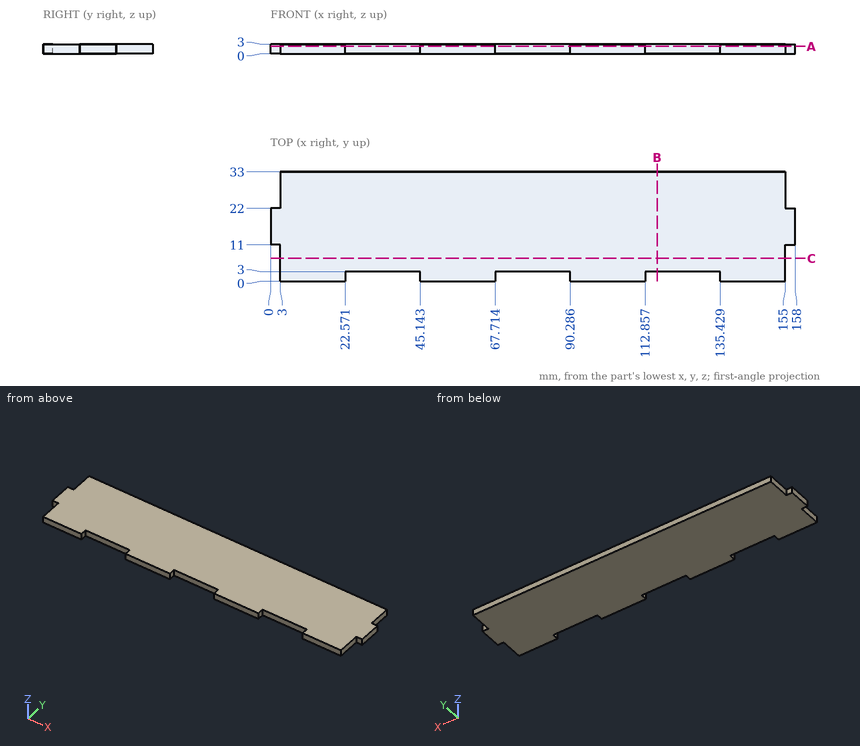
Drawing for the job (mm, zero at the part's lowest x, y, z). Round coordinates to 2 decimals unless told otherwise and drop trailing zeros. Order: outer loops, then holes, each group sorted by start corner. A loop starts at its lowest first (then second) coordinate and runs counter-clockwise, first axis right, second up. Notation, with made-up numbers: (87.5, 54.25) -> (96.5, 54.25) arc R13 cw to (96.5, 68.25) -> close; hole circle Ø9 at (81, 28.25). An arc over 180 degrees is marked (long way). Put each result on its own line as item: value.
Q1. Band-saw the part on C-C (y = 7). Give the cut face in (x, z).
From the geometry:
outline: (3, 0) -> (155, 0) -> (155, 3) -> (3, 3) -> close
Q2. Wall check: line 1 (X direction, y = 2, z = 2.8) (1 decimal); line 2 (Y direction, x = 85.5, z = 2); line 3 (X direction, y = 7, z = 2.6). Give the ranges that are in metal, low to high. Write a range as [from, to].
From the geometry:
line 1: x = [3, 22.6], [45.1, 67.7], [90.3, 112.9], [135.4, 155]
line 2: y = [3, 33]
line 3: x = [3, 155]
Q3. Band-saw the part on A-A (z = 2.3). Give the cut face in (x, y) (1 decimal), and give its area (3 significant figures).
From the geometry:
outline: (0, 11) -> (3, 11) -> (3, 0) -> (22.6, 0) -> (22.6, 3) -> (45.1, 3) -> (45.1, 0) -> (67.7, 0) -> (67.7, 3) -> (90.3, 3) -> (90.3, 0) -> (112.9, 0) -> (112.9, 3) -> (135.4, 3) -> (135.4, 0) -> (155, 0) -> (155, 11) -> (158, 11) -> (158, 22) -> (155, 22) -> (155, 33) -> (3, 33) -> (3, 22) -> (0, 22) -> close
area: 4,880 mm2
Q4. Pin check, flat tips, straight feed: pin 1 Ø0.9 at (x, z) = (38, 1.5) entering from -Y; pin 2 Ø0.9 at (x, z) = (2, 1.5) entering from -Y; pin 3 Ø0.9 at (y, z) = (2, 1) entering from -X; pin 4 Ø4 at (x, y) = (101, 15) entering from -Z. Stop position of each tip, or through.
From the geometry:
pin 1: stops at y = 3
pin 2: stops at y = 11
pin 3: stops at x = 3
pin 4: stops at z = 0
Q5. Band-saw the part on B-B (x = 116.5). Give the cut face in (y, z).
From the geometry:
outline: (3, 0) -> (33, 0) -> (33, 3) -> (3, 3) -> close
